Read the model definition and answer for the solid it produces. Units are mm, in the model's axes. A direction names the side the tool comes from. Give positions to 0.01 mm unless a question says otherwise; leave off trailing zeros. Loops run counter-clockwise (first coordinate to the right, second up) from the corner with the lowest first, then second, coordinate; pieces in that order, holes last. Notation, with made-up numbers: (7.5, 25.25) - (20.5, 25.25) arc R23 cw to (20.5, 48.25) - close; hole circle Ø10 at (-31.75, -26.75). An arc over 180 degrees is marked (long way). Use a Markdown table: item, result. Add a question column.
Item 1: A cutting plane is placed at A-A (y = 2.5). Determine the outline of the cut face in (x, z) (3 decimals), plus the area to 3 significant figures.
Item 2: For a pull along Z with two mould halves and no side action, classify faces 1 (the face through (-13.557, 1.565, -1.565)), 2 (the face through (-7, 0, 6.35)), 3 (the face through (-6, 0, -6.35)), 4 (the face through (-9.31, -1.57, -0.2)) as +Z half, -Z half, draft (parallel to the pull), parting line (faces both ways), or undercut.
Item 3: Consider probe 1 along X at (y, z) = (-1, 0) (3 decimals); probe 2 along Z at (x, y) = (-15, 2.5); probe 3 along X at (y, z) = (-2, -14) (3 decimals). Determine where each line is inside the solid, lowest interval first. Write a range as [from, to].
Item 4: Which of the six approach directions +Z, -Z, +X, -X, +Y, -Y give full straight-line access (tool end or side, diameter ignored) to faces 5 (the face through (4.445, -2, 18)), 6 (the face through (4.445, -2, -22)), 7 (the face through (11, 0, -4)), 8 (the face through (-11, 2, 3.175)), 9 (the face through (11, -2, -36.83))?
Item 5: A cutting plane is placed at B-B (z = 20). Determine the outline of the cut face in (x, y) (3 decimals).
Item 6: Each of these flat-tipped pins is pushed along its axis until it touches: P1, Ø3.5, axis at x = -10, y = 1, coming from the +Z side; P2, Ø2.5, axis at y = 2, z = -2, coming from the +X side (3 decimals); P3, Ø1, axis at y = -1, z = -21, coming from the -X side (3 decimals); P4, Ø1, axis at y = 1, z = -7, coming from the +X side. Where does it stop, or does it pass through?
Item 7: A cutting plane is placed at C-C (y = -1.5). Determine the outline of the cut face in (x, z) (3 decimals), plus the area to 3 significant figures.
from build123d import *

# Parameters (mm, degrees)
SKETCH1_W           = 21.59
SKETCH1_H           = 12.7
BOSS_EXTRUDE3_DEPTH = 3.175
SKETCH1_5_R         = 1.5
BOSS_EXTRUDE4_DEPTH = 3.175


with BuildPart() as part:
    # Sketch1 → Boss-Extrude3 (new body)
    with BuildSketch(Plane(origin=(0, 0, 0), x_dir=(1, 0, 0), z_dir=(0, 1, 0))):
        with Locations((-6.35, 0)):
            Rectangle(SKETCH1_W, SKETCH1_H)
        Polygon((-7.128825791, 0), (-8.961912895, -3.175), (-12.628087105, -3.175), (-14.461174209, 0), (-12.628087105, 3.175), (-8.961912895, 3.175), align=None, mode=Mode.SUBTRACT)
    extrude(amount=BOSS_EXTRUDE3_DEPTH)

    # Sketch1_5 → Boss-Extrude4 (add)
    with BuildSketch(Plane(origin=(0, 0, 0), x_dir=(1, 0, 0), z_dir=(0, 1, 0))):
        Polygon((17.145, -29.52), (17.145, 36.83), (4.445, 36.83), (4.445, 6.35), (-17.145, 6.35), (-17.145, -6.35), (4.445, -6.35), (4.445, -29.52), align=None)
        with Locations(Location((-10.795, 0, 0), (0, 0, 270))):
            Circle(SKETCH1_5_R, mode=Mode.SUBTRACT)
    extrude(amount=-BOSS_EXTRUDE4_DEPTH)


solid = part.part
Geometry says:
| question | item | result |
|---|---|---|
| 1 | outline | (-17.145, -6.35) - (4.445, -6.35) - (4.445, 6.35) - (-17.145, 6.35) - close; hole (-14.461, 0) - (-12.628, -3.175) - (-8.962, -3.175) - (-7.129, 0) - (-8.962, 3.175) - (-12.628, 3.175) - close |
| 1 | area | 239 mm² |
| 2 | face 1 | undercut |
| 2 | face 2 | +Z half |
| 2 | face 3 | -Z half |
| 2 | face 4 | undercut |
| 3 | probe 1 | [-17.145, -12.295], [-9.295, 17.145] |
| 3 | probe 2 | [-6.35, 6.35] |
| 3 | probe 3 | [4.445, 17.145] |
| 4 | face 5 | +Z, -X, +Y, -Y |
| 4 | face 6 | -Z, -X, +Y, -Y |
| 4 | face 7 | +Z, -Z, +X, +Y |
| 4 | face 8 | +Y |
| 4 | face 9 | -Z, +X, -X, +Y, -Y |
| 5 | outline | (4.445, -3.175) - (17.145, -3.175) - (17.145, 0) - (4.445, 0) - close |
| 6 | P1 | z = 6.35 |
| 6 | P2 | x = 4.445 |
| 6 | P3 | x = 4.445 |
| 6 | P4 | through |
| 7 | outline | (-17.145, -6.35) - (4.445, -6.35) - (4.445, -36.83) - (17.145, -36.83) - (17.145, 29.52) - (4.445, 29.52) - (4.445, 6.35) - (-17.145, 6.35) - close; hole circle Ø3 at (-10.795, 0) |
| 7 | area | 1,110 mm² |
